```python
from build123d import *

# Parameters (mm, degrees)
F1_DEPTH = 7
F4_DEPTH = 25
F5_DEPTH = 25
F6_DEPTH = 25
F7_COUNT = 3
F8_DEPTH = 7


# Not quite as in the source:
# - a feature names something its author has since deleted; it is built from what else it names


with BuildPart() as f1:
    # F0 (on Top) → F1 (new body)
    with BuildSketch(Plane.XY):
        with BuildLine():
            ThreePointArc((-13.7992422924, -9.0114684358), (-14.4938657477, 7.8456043045), (0, 16.4810694803))
            ThreePointArc((0, 16.4810694803), (-14.068080809, 30.8723339162), (-6.2153203117, 49.4021353799))
            Line((-6.2153203117, 49.4021353799), (-2.3028528943, 51.9794964298))
            Line((-2.3028528943, 51.9794964298), (-7.0776391154, 51.2091623618))
            ThreePointArc((-7.0776391154, 51.2091623618), (-31.8683563703, 23.4907745685), (-13.7992422924, -9.0114684358))
        make_face()
    extrude(amount=F1_DEPTH)

    # F2 (on Top) → F4 (cut)
    with BuildSketch(Plane.XY):
        with BuildLine():
            ThreePointArc((-19.9399101365, 36.2145881717), (-17.5331910144, 36.3619404524), (-16.370389089, 38.4742617607))
            ThreePointArc((-16.370389089, 38.4742617607), (-16.6966666914, 39.7091427016), (-17.5903338395, 40.6216924484))
            ThreePointArc((-17.5903338395, 40.6216924484), (-18.870389089, 38.4742617607), (-19.9399101365, 36.2145881717))
        make_face()
        with BuildLine():
            ThreePointArc((-12.9184592818, 14.9145969957), (-15.6103285505, 20.1822473574), (-21.4563486152, 21.0868742954))
            ThreePointArc((-21.4563486152, 21.0868742954), (-19.4184592818, 14.9145969957), (-15.9236151324, 9.4340801978))
            ThreePointArc((-15.9236151324, 9.4340801978), (-13.7190519893, 11.7894159586), (-12.9184592818, 14.9145969957))
        make_face()
        with BuildLine():
            ThreePointArc((-15.9236151324, 9.4340801978), (-19.4184592818, 14.9145969957), (-21.4563486152, 21.0868742954))
            ThreePointArc((-21.4563486152, 21.0868742954), (-25.2902206788, 12.1266913129), (-15.9236151324, 9.4340801978))
        make_face()
        with BuildLine():
            ThreePointArc((-17.3422204011, 28.5281271909), (-18.3916105886, 31.4166028999), (-21.0503501441, 32.9579061352))
            ThreePointArc((-21.0503501441, 32.9579061352), (-21.8422204011, 28.5281271909), (-21.8642642373, 24.0281811835))
            ThreePointArc((-21.8642642373, 24.0281811835), (-18.6680431268, 25.3383625238), (-17.3422204011, 28.5281271909))
        make_face()
        with BuildLine():
            ThreePointArc((-21.8642642373, 24.0281811835), (-21.8422204011, 28.5281271909), (-21.0503501441, 32.9579061352))
            ThreePointArc((-21.0503501441, 32.9579061352), (-26.3236437362, 28.9365937035), (-21.8642642373, 24.0281811835))
        make_face()
        with BuildLine():
            ThreePointArc((-19.9399101365, 36.2145881717), (-18.870389089, 38.4742617607), (-17.5903338395, 40.6216924484))
            ThreePointArc((-17.5903338395, 40.6216924484), (-21.0764541807, 39.6503896496), (-19.9399101365, 36.2145881717))
        make_face()
    extrude(amount=-F4_DEPTH, mode=Mode.SUBTRACT)

    # F2 (on Top) → F5 (cut)
    with BuildSketch(Plane.XY):
        with BuildLine():
            ThreePointArc((-19.9399101365, 36.2145881717), (-17.5331910144, 36.3619404524), (-16.370389089, 38.4742617607))
            ThreePointArc((-16.370389089, 38.4742617607), (-16.6966666914, 39.7091427016), (-17.5903338395, 40.6216924484))
            ThreePointArc((-17.5903338395, 40.6216924484), (-18.870389089, 38.4742617607), (-19.9399101365, 36.2145881717))
        make_face()
        with BuildLine():
            ThreePointArc((-12.9184592818, 14.9145969957), (-15.6103285505, 20.1822473574), (-21.4563486152, 21.0868742954))
            ThreePointArc((-21.4563486152, 21.0868742954), (-19.4184592818, 14.9145969957), (-15.9236151324, 9.4340801978))
            ThreePointArc((-15.9236151324, 9.4340801978), (-13.7190519893, 11.7894159586), (-12.9184592818, 14.9145969957))
        make_face()
        with BuildLine():
            ThreePointArc((-15.9236151324, 9.4340801978), (-19.4184592818, 14.9145969957), (-21.4563486152, 21.0868742954))
            ThreePointArc((-21.4563486152, 21.0868742954), (-25.2902206788, 12.1266913129), (-15.9236151324, 9.4340801978))
        make_face()
        with BuildLine():
            ThreePointArc((-17.3422204011, 28.5281271909), (-18.3916105886, 31.4166028999), (-21.0503501441, 32.9579061352))
            ThreePointArc((-21.0503501441, 32.9579061352), (-21.8422204011, 28.5281271909), (-21.8642642373, 24.0281811835))
            ThreePointArc((-21.8642642373, 24.0281811835), (-18.6680431268, 25.3383625238), (-17.3422204011, 28.5281271909))
        make_face()
        with BuildLine():
            ThreePointArc((-21.8642642373, 24.0281811835), (-21.8422204011, 28.5281271909), (-21.0503501441, 32.9579061352))
            ThreePointArc((-21.0503501441, 32.9579061352), (-26.3236437362, 28.9365937035), (-21.8642642373, 24.0281811835))
        make_face()
        with BuildLine():
            ThreePointArc((-19.9399101365, 36.2145881717), (-18.870389089, 38.4742617607), (-17.5903338395, 40.6216924484))
            ThreePointArc((-17.5903338395, 40.6216924484), (-21.0764541807, 39.6503896496), (-19.9399101365, 36.2145881717))
        make_face()
    extrude(amount=-F5_DEPTH, mode=Mode.SUBTRACT)

    # F2 (on Top) → F6 (cut)
    with BuildSketch(Plane.XY):
        with BuildLine():
            ThreePointArc((-19.9399101365, 36.2145881717), (-17.5331910144, 36.3619404524), (-16.370389089, 38.4742617607))
            ThreePointArc((-16.370389089, 38.4742617607), (-16.6966666914, 39.7091427016), (-17.5903338395, 40.6216924484))
            ThreePointArc((-17.5903338395, 40.6216924484), (-18.870389089, 38.4742617607), (-19.9399101365, 36.2145881717))
        make_face()
        with BuildLine():
            ThreePointArc((-12.9184592818, 14.9145969957), (-15.6103285505, 20.1822473574), (-21.4563486152, 21.0868742954))
            ThreePointArc((-21.4563486152, 21.0868742954), (-19.4184592818, 14.9145969957), (-15.9236151324, 9.4340801978))
            ThreePointArc((-15.9236151324, 9.4340801978), (-13.7190519893, 11.7894159586), (-12.9184592818, 14.9145969957))
        make_face()
        with BuildLine():
            ThreePointArc((-15.9236151324, 9.4340801978), (-19.4184592818, 14.9145969957), (-21.4563486152, 21.0868742954))
            ThreePointArc((-21.4563486152, 21.0868742954), (-25.2902206788, 12.1266913129), (-15.9236151324, 9.4340801978))
        make_face()
        with BuildLine():
            ThreePointArc((-17.3422204011, 28.5281271909), (-18.3916105886, 31.4166028999), (-21.0503501441, 32.9579061352))
            ThreePointArc((-21.0503501441, 32.9579061352), (-21.8422204011, 28.5281271909), (-21.8642642373, 24.0281811835))
            ThreePointArc((-21.8642642373, 24.0281811835), (-18.6680431268, 25.3383625238), (-17.3422204011, 28.5281271909))
        make_face()
        with BuildLine():
            ThreePointArc((-21.8642642373, 24.0281811835), (-21.8422204011, 28.5281271909), (-21.0503501441, 32.9579061352))
            ThreePointArc((-21.0503501441, 32.9579061352), (-26.3236437362, 28.9365937035), (-21.8642642373, 24.0281811835))
        make_face()
        with BuildLine():
            ThreePointArc((-19.9399101365, 36.2145881717), (-18.870389089, 38.4742617607), (-17.5903338395, 40.6216924484))
            ThreePointArc((-17.5903338395, 40.6216924484), (-21.0764541807, 39.6503896496), (-19.9399101365, 36.2145881717))
        make_face()
    extrude(amount=F6_DEPTH, mode=Mode.SUBTRACT)


with BuildPart() as f7_1:
    # F7: instance of F1
    add(f1.part.rotate(Axis((0, 0, -1.6987677664), (0, 0, -1)), 1 * 360 / F7_COUNT))


with BuildPart() as f7_2:
    # F7: instance of F1
    add(f1.part.rotate(Axis((0, 0, -1.6987677664), (0, 0, -1)), 2 * 360 / F7_COUNT))


with BuildPart() as f1_1:
    add(f1.part)

    add(f7_1.part)  # F8 merges F7_1

    add(f7_2.part)  # F8 merges F7_2
    # F0 (on Top) → F8 (join)
    with BuildSketch(Plane.XY):
        with BuildLine():
            Line((0, 16.4810694803), (0, 11.5))
            ThreePointArc((0, 11.5), (8.1317279836, 8.1317279836), (11.5, 0))
            ThreePointArc((11.5, 0), (3.2802394095, -11.0222515584), (-9.628700768, -6.2879345989))
            Line((-9.628700768, -6.2879345989), (-13.7992422924, -9.0114684358))
            ThreePointArc((-13.7992422924, -9.0114684358), (4.7010307496, -15.796390762), (16.4810694803, 0))
            ThreePointArc((16.4810694803, 0), (11.6538759907, 11.6538759907), (0, 16.4810694803))
        make_face()
        with BuildLine():
            ThreePointArc((-9.628700768, -6.2879345989), (-10.1133883513, 5.4744292905), (0, 11.5))
            Line((0, 11.5), (0, 16.4810694803))
            ThreePointArc((0, 16.4810694803), (-14.4938657477, 7.8456043045), (-13.7992422924, -9.0114684358))
            Line((-13.7992422924, -9.0114684358), (-9.628700768, -6.2879345989))
        make_face()
    extrude(amount=F8_DEPTH)


solid = f1_1.part
```
Input: part model. Units: mm. Frame: model coordinates. A direction names the side the tool comes from. Give positions to 0.01 mm unless a question says otherwise; leave off trailing zeros. Loops run counter-clockwise (first coordinate to the right, second up) from the corner with the lowest first, then second, coordinate; pieces in that order, holes last. Notation, with made-up numbers: (-2, 29.25) -> (3, 29.25) arc R28 cw to (3, 54.25) -> close; hole circle Ø4 at (11, -14.75). An arc over 180 degrees is marked (long way). Use a Markdown table: item, result.
Q1. Section query A-A, the plane y = 31. Return the cut outline in (x, z), plus the area to 3 significant figures.
Entries:
| item | result |
|---|---|
| outline | (-30.1, 0) -> (-25.6, 0) -> (-25.6, 7) -> (-30.1, 7) -> close; (-18.08, 0) -> (-14.09, 0) -> (-14.09, 7) -> (-18.08, 7) -> close |
| area | 59.4 mm² |
Q2. Section query C-C, the plane x = -24. Return the cut outline in (y, z), plus the area to 3 significant figures.
Entries:
| item | result |
|---|---|
| outline | (-41.32, 0) -> (-38.08, 0) -> (-38.08, 7) -> (-41.32, 7) -> close; (-33.08, 0) -> (-30.37, 0) -> (-30.37, 7) -> (-33.08, 7) -> close; (-1.33, 0) -> (10.3, 0) -> (10.3, 7) -> (-1.33, 7) -> close; (19.53, 0) -> (24.58, 0) -> (24.58, 7) -> (19.53, 7) -> close; (32.48, 0) -> (41.2, 0) -> (41.2, 7) -> (32.48, 7) -> close |
| area | 220 mm² |
Q3. Section query B-B, the plane x = -4. Return the cut outline in (y, z).
Entries:
| item | result |
|---|---|
| outline | (-39.16, 0) -> (-30.73, 0) -> (-30.73, 7) -> (-39.16, 7) -> close; (-17.82, 0) -> (-10.78, 0) -> (-10.78, 7) -> (-17.82, 7) -> close; (10.78, 0) -> (17.83, 0) -> (17.83, 7) -> (10.78, 7) -> close; (50.86, 0) -> (51.71, 0) -> (51.71, 7) -> (50.86, 7) -> close |
Q4. First-contact query: P1, Ø17, axis at x = -19.42, y = 14.91, coming from the -Z side; P2, Ø1.5, axis at y = 31.5, z = 2.5, coming from the -X side. Flat tips, straight axial feed; report the tip coordinate or a pass-through.
Entries:
| item | result |
|---|---|
| P1 | stops at z = 0 |
| P2 | stops at x = -30.19 |
Q5. Access query for faces 1 (the flat face through (-4.29, 50.67, 3.45)), 2 (the flat face through (46.027, -21.624, 3.451)), 3 (the cylindrical face through (-31.782, 24.194, 3.451)), 4 (the flat face through (-41.74, -29.05, 3.45)). Directions: +Z, -Z, +X, -X, +Y, -Y. A direction counts if a zero-diameter tool reaches every point of the face in a straight line with its end or side. Return the directions, or none.
Entries:
| item | result |
|---|---|
| face 1 | +Z, -Z, +X |
| face 2 | +Z, -Z, -Y |
| face 3 | +Z, -Z, -X |
| face 4 | +Z, -Z, +Y |
Q6. Ray query, probe 1 along X at (y, z) = (1.5, 0.75); probe 2 along Y at (x, z) = (-21, 6.5); probe 3 along X at (y, z) = (-4, 2.75). Return the intervals inside material, ascending. Write a range as from..to.
Entries:
| item | result |
|---|---|
| probe 1 | x = -26.24..-11.4, 11.4..32.42, 38.84..47.21 |
| probe 2 | y = -41.81..-28.64, -4.3..8.61, 21.22..24.11, 32.95..37.16, 39.78..44.17 |
| probe 3 | x = -21.34..-10.78, 10.78..19.95, 35.58..40.51, 45..48.77 |
Q7. Section query D-D, the plane y = -16.5. Return the cut outline in (x, z), plus the area to 3 significant figures.
Entries:
| item | result |
|---|---|
| outline | (-13.58, 0) -> (14.13, 0) -> (14.13, 7) -> (-13.58, 7) -> close; (45.5, 0) -> (48.66, 0) -> (48.66, 7) -> (45.5, 7) -> close |
| area | 216 mm² |
Q8. Pull-direction query (X, two-part tool) for faces 5 (the flat face through (-4.66, 51.6, 3.45)), 6 (the cylindrical face through (-19.731, -27.644, 3.451)), 7 (the cylindrical face through (-14.075, 30.91, 3.451)), 8 (the flat face through (47.015, -21.767, 3.451)); classes: pulls with the +X half, pulls with the -X half, needs draft (parallel to the pull), parting line crosses it, or undercut.
Entries:
| item | result |
|---|---|
| face 5 | pulls with the -X half |
| face 6 | undercut |
| face 7 | undercut |
| face 8 | pulls with the +X half |
